Geometry check sheet. Reference: the model listing, model coordinates, mm. Face numbers are marked on the shaded views. A direction names the side the tool comes from. Round coordinates to 2 decimals unless told otherwise and drop trailing zeros. Order: outer loops, then holes, each group sorted by start corner. A loop starts at its lowest first (then second) coordinate and runs counter-clockwise, first axis right, second up.
(1) Cross-section at C-C on x = 13.5. Count the separate pieces of the cut face and the enclosed holes in it, and give its area (3 significant figures).
(2) Gauge pin test, flat ends, axial feed: P1, Ø4, axis at x = 2.5, y = 15.5, coming from the -Z side; P2, Ø2, axis at x = 13.5, z = -6.5, coming from the -Y side; P3, Ø4, axis at x = 14, z = 0, coming from the +Y side. Record the tip position at first contact, or that the pin passes through.
(3) Thickness scan on L1, parallel to Z at x = 13.5, y = 2.2; L2, parallel to X at y = 0.8, z = -6.5; L3, parallel to Y at x = 13.5, z = 8.1. Record the ranges inside material, lowest first.
(4) Cross-section at D-D on x = 4. Enter the section's corners in (y, z), and give its area (3 significant figures).
(5) Set-up check for the marked faces 1 and 2: record each of +Z, -Z, +X, -X, +Y, -Y from which the full face is reachable in a straight line by a thin tool's end or side.
(6) Draft check along Z on the marked faces 3, 4, 5 and 6. Enter one of: pulls with the +Z half, pulls with the -Z half, needs draft (parallel to the pull), parting line crosses it, or undercut.
(7) Cross-section at A-A on z = 0.5. Enter the section's corners in (x, y) (3 decimals).
(8) Cross-section at B-B on y = 16.5. Enter the section's corners in (x, z) (3 decimals), and give its area (3 significant figures).
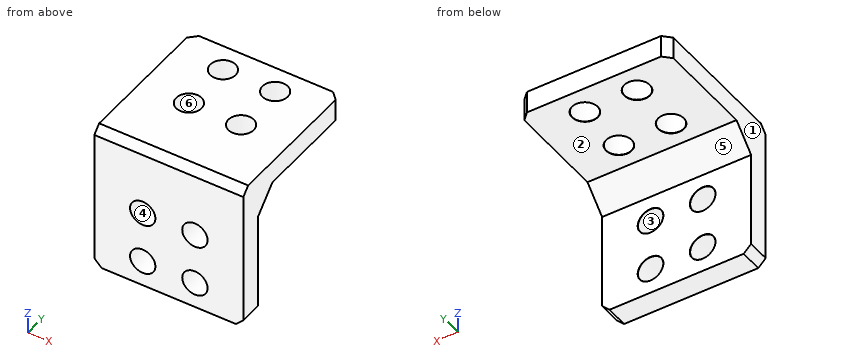
from build123d import *

# Parameters (mm, degrees)
EXTRUDE_THIN1_DEPTH            = 20
CHAMFER1_SIZE                  = 3
M3_CLEARANCE_HOLE1_D           = 3.4
M3_CLEARANCE_HOLE1_DEPTH       = 6
M3_CLEARANCE_HOLE1_CSINK_D     = 3.45
M3_CLEARANCE_HOLE1_CSINK_ANGLE = 90
M3_CLEARANCE_HOLE1_TIP         = 1.021463052
CHAMFER2_SIZE                  = 1


# Read off the part's stored shape, not the designer's step: M3 Clearance Hole2
with BuildPart() as part:
    # Sketch2 → Extrude-Thin1 (new body)
    with BuildSketch(Plane(origin=(0, 0, 0), x_dir=(0, 0, -1), z_dir=(1, 0, 0))):
        Polygon((-10, 20), (-10, 0), (10, 0), (10, 3), (-7, 3), (-7, 20), align=None)
    extrude(amount=EXTRUDE_THIN1_DEPTH)

    # Chamfer1
    chamfer1_edges = [part.edges().sort_by_distance(p)[0] for p in [
        (10, 3, 7),
    ]]
    chamfer(chamfer1_edges, length=CHAMFER1_SIZE)

    # M3 Clearance Hole1
    with Locations(Plane(origin=(0, 3, 0), x_dir=(1, 0, 0), z_dir=(0, 1, 0))):
        with Locations((6.5, 6.5), (13.5, 6.5), (13.5, -0.5), (6.5, -0.5)):
            CounterSinkHole(M3_CLEARANCE_HOLE1_D / 2, M3_CLEARANCE_HOLE1_CSINK_D / 2, depth=M3_CLEARANCE_HOLE1_DEPTH, counter_sink_angle=M3_CLEARANCE_HOLE1_CSINK_ANGLE)
            with Locations((0, 0, -(M3_CLEARANCE_HOLE1_DEPTH + M3_CLEARANCE_HOLE1_TIP / 2))):  # 118° drill point
                Cone(0, M3_CLEARANCE_HOLE1_D / 2, M3_CLEARANCE_HOLE1_TIP, mode=Mode.SUBTRACT)

    # M3 Clearance Hole2 outline → M3 Clearance Hole2 (revolve, cut)
    with BuildSketch(Plane(origin=(6.5, 9.5, 0), x_dir=(1, 0, 0), z_dir=(0, -1, 0))):
        Polygon((1.7, 7.025), (1.7, 10), (0, 10), (0, 7), (1.725, 7), align=None)
    revolve(axis=Axis((6.5, 9.5, 0), (0, 0, 1)), mode=Mode.SUBTRACT)

    # M3 Clearance Hole2 2 outline → M3 Clearance Hole2 2 (revolve, cut)
    with BuildSketch(Plane(origin=(13.5, 16.5, 0), x_dir=(1, 0, 0), z_dir=(0, -1, 0))):
        Polygon((1.7, 7.025), (1.7, 10), (0, 10), (0, 7), (1.725, 7), align=None)
    revolve(axis=Axis((13.5, 16.5, 0), (0, 0, 1)), mode=Mode.SUBTRACT)

    # M3 Clearance Hole2 3 outline → M3 Clearance Hole2 3 (revolve, cut)
    with BuildSketch(Plane(origin=(13.5, 9.5, 0), x_dir=(1, 0, 0), z_dir=(0, -1, 0))):
        Polygon((1.7, 7.025), (1.7, 10), (0, 10), (0, 7), (1.725, 7), align=None)
    revolve(axis=Axis((13.5, 9.5, 0), (0, 0, 1)), mode=Mode.SUBTRACT)

    # M3 Clearance Hole2 4 outline → M3 Clearance Hole2 4 (revolve, cut)
    with BuildSketch(Plane(origin=(6.5, 16.5, 0), x_dir=(1, 0, 0), z_dir=(0, -1, 0))):
        Polygon((1.7, 7.025), (1.7, 10), (0, 10), (0, 7), (1.725, 7), align=None)
    revolve(axis=Axis((6.5, 16.5, 0), (0, 0, 1)), mode=Mode.SUBTRACT)

    # Chamfer2
    chamfer2_edges = [part.edges().sort_by_distance(p)[0] for p in [
        (20, 1.5, -10),
        (0, 1.5, -10),
        (0, 20, 8.5),
        (20, 20, 8.5),
        (10, 0, 10),
    ]]
    chamfer(chamfer2_edges, length=CHAMFER2_SIZE)


solid = part.part
Found:
1. separate pieces: 5
1. enclosed holes: 0
1. area: 74.2 mm2
2. P1: stops at z = 7
2. P2: passes through
2. P3: stops at y = 3
3. L1: z = -10 to -8.2, -4.8 to -1.2, 2.2 to 10
3. L2: x = 0 to 4.8, 8.2 to 11.8, 15.2 to 20
3. L3: y = 0 to 7.8, 11.2 to 14.8, 18.2 to 20
4. outline: (0, -10) - (3, -10) - (3, 4) - (6, 7) - (20, 7) - (20, 10) - (1, 10) - (0, 9) - close
4. area: 115 mm2
5. face 1: +Z, -Z, -X, +Y, -Y
5. face 2: -Z, +X, -X, +Y
6. face 3: undercut
6. face 4: undercut
6. face 5: pulls with the -Z half
6. face 6: needs draft
7. outline: (0, 0) - (4.8, 0) - (4.8, 2.975) - (4.775, 3) - (0, 3) - close; (8.2, 0) - (11.8, 0) - (11.8, 2.975) - (11.775, 3) - (8.225, 3) - (8.2, 2.975) - close; (15.2, 0) - (20, 0) - (20, 3) - (15.225, 3) - (15.2, 2.975) - close
8. outline: (0, 7) - (4.775, 7) - (4.8, 7.025) - (4.8, 10) - (0, 10) - close; (8.2, 7.025) - (8.225, 7) - (11.775, 7) - (11.8, 7.025) - (11.8, 10) - (8.2, 10) - close; (15.2, 7.025) - (15.225, 7) - (20, 7) - (20, 10) - (15.2, 10) - close
8. area: 39.6 mm2
